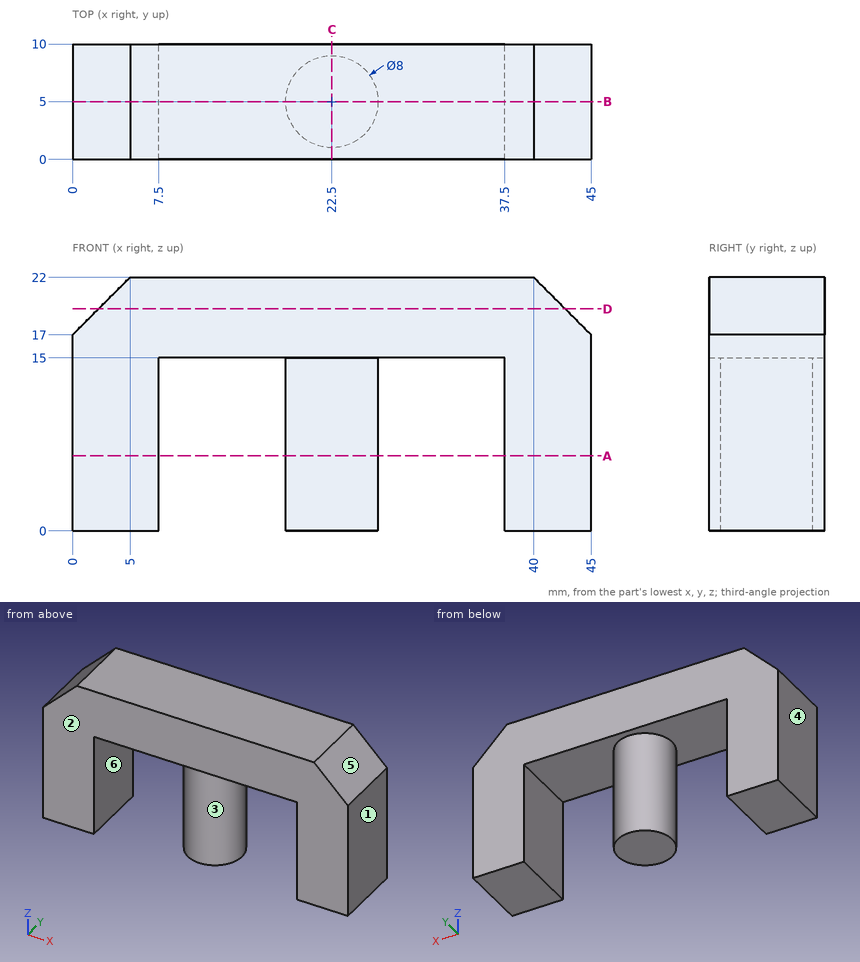
The drawing under review shows one solid part. Ordinate dimensions are in mm from its lowest x, y, z. A direction names the side the tool comes from. Coordinates: 2 decimals unless noted, no trailing zeros. Write each loop counter-clockwise with the first axis right and the second up, starting at its lowest first coordinate (ties: lowest second). Pieces come first, ordered by that corner, then holes. Notation, with made-up numbers: (14.5, 75.25) - (48.5, 75.25) arc R16 cw to (48.5, 88.25) - close; hole circle Ø3 at (31, 59). An arc over 180 degrees is marked (long way). Answer as CSV lines item,"result".
(1) We need section D-D (z = 19.25). Give the boundary of the cut face in (x, y).
Data:
outline,"(2.25, 0) - (42.75, 0) - (42.75, 10) - (2.25, 10) - close"
(2) We need section A-A (z = 6.5). Give the boundary of the cut face in (x, y).
Data:
outline,"(0, 0) - (7.5, 0) - (7.5, 10) - (0, 10) - close; circle Ø8 at (22.5, 5); (37.5, 0) - (45, 0) - (45, 10) - (37.5, 10) - close"
(3) Tool access review of the marked faces 5 and 6: name each direction out of +Z, -Z, +X, -X, +Y, -Y from which nothing blocks a thin tool from reaching the whole face with its end or side.
Data:
face 5,"+Z, +X, +Y, -Y"
face 6,"-Z, +Y, -Y"
(4) Clearance check with a flat-ended pin moving along its axis: pin 1 Ø1.5 at (x, z) = (16, 5) entering from -Y. State where the tip first meets the part, or that it passes through.
Data:
pin 1,"passes through"
(5) We need section B-B (y = 5). Give the boundary of the cut face in (x, z).
Data:
outline,"(0, 0) - (7.5, 0) - (7.5, 15) - (18.5, 15) - (18.5, 0) - (26.5, 0) - (26.5, 15) - (37.5, 15) - (37.5, 0) - (45, 0) - (45, 17) - (40, 22) - (5, 22) - (0, 17) - close"
(6) We need section C-C (x = 22.5). Give the boundary of the cut face in (y, z).
Data:
outline,"(0, 15) - (1, 15) - (1, 0) - (9, 0) - (9, 15) - (10, 15) - (10, 22) - (0, 22) - close"
(7) Mouldability with a two-part tool opening along X and no side actions: class the marked faces 1, 2, 3 and 4 as pulls with the +X half, pulls with the -X half, needs draft (parallel to the pull), parting line crosses it, or undercut.
Data:
face 1,"pulls with the +X half"
face 2,"needs draft"
face 3,"undercut"
face 4,"pulls with the -X half"
(8) For line 1 along X through (y, z) = (5, 5.75); line 2 along X through (y, z) = (9.25, 9.25); line 3 along X through (y, z) = (1.5, 7.75), list the stretches that pass through material, from the lowest coordinate up. Write a range as [from, to].
Data:
line 1,"x = [0, 7.5], [18.5, 26.5], [37.5, 45]"
line 2,"x = [0, 7.5], [37.5, 45]"
line 3,"x = [0, 7.5], [20.56, 24.44], [37.5, 45]"
